from build123d import *

# Parameters (mm, degrees)
REVOLVE_2_ANGLE     = 180
EXTRUDE_3_REACH     = 142.262
SKETCH_1_12_R       = 4.474143501
CUT_EXTRUDE_3_DEPTH = 204.9
SKETCH_1_14_R       = 4.474143501
EXTRUDE_4_DEPTH     = 10
SKETCH_1_16_R       = 3
CUT_EXTRUDE_4_DEPTH = 32


with BuildPart() as part:
    # Sketch 1 → Revolve 2 (revolve)
    with BuildSketch(Plane.XY):
        Polygon((14, 48.5), (10, 48.5), (10, 32), (7, 32), (7, 35), (0, 35), (0, 51), (14, 51), (14, 52.5), (53.673378029, 34), (119, 34), (119, 32), (53.673378029, 32), align=None)
    revolve(axis=Axis((0, 0, 0), (1, 0, 0)), revolution_arc=REVOLVE_2_ANGLE)

    # Sketch 1_11 → Extrude 3 (add, up to next)
    with BuildSketch(Plane.XY, mode=Mode.PRIVATE) as extrude_3_sk1:
        Polygon((25, 43.925143786), (25, 32), (35, 32), (35, 39.766183592), align=None)
    extrude_3_tool1 = extrude(extrude_3_sk1.sketch, amount=EXTRUDE_3_REACH, mode=Mode.PRIVATE) - part.part
    extrude_3 = extrude_3_tool1.solids().sort_by_distance((29.647987, 36.996032, 0))[0]
    add(extrude_3)

    # Sketch 1_12 → Cut-Extrude 3 (cut)
    with BuildSketch(Plane.XY):
        with Locations(Location((30, 37, 0), (0, 0, 38.236616633))):
            Circle(SKETCH_1_12_R)
    cut_extrude_3 = extrude(amount=CUT_EXTRUDE_3_DEPTH, mode=Mode.SUBTRACT)

    # Sketch 1_14 → Extrude 4 (add)
    with BuildSketch(Plane.XY):
        with Locations(Location((30, 37, 0), (0, 0, 38.236616633))):
            Circle(SKETCH_1_14_R)
    extrude_4 = extrude(amount=EXTRUDE_4_DEPTH)

    # Sketch 1_16 → Cut-Extrude 4 (cut)
    with BuildSketch(Plane.XY):
        with Locations((30, 37)):
            Circle(SKETCH_1_16_R)
    cut_extrude_4 = extrude(amount=CUT_EXTRUDE_4_DEPTH, mode=Mode.SUBTRACT)

    # Mirror 1: Extrude 3, Cut-Extrude 3, Extrude 4, Cut-Extrude 4 across plane
    add(extrude_3.mirror(Plane.ZX))
    add(cut_extrude_3.mirror(Plane.ZX), mode=Mode.SUBTRACT)
    add(extrude_4.mirror(Plane.ZX))
    add(cut_extrude_4.mirror(Plane.ZX), mode=Mode.SUBTRACT)


solid = part.part
CAD build for the part. Positions are in the model's coordinates, mm. A direction names the side the tool comes from. Give positions to 0.01 mm unless a question says otherwise; leave off trailing zeros. Loops run counter-clockwise (first coordinate to the right, second up) from the corner with the lowest first, then second, coordinate; pieces in that order, holes last. Notation, with made-up numbers: M 23.25,-17 L 65.25,-17 A30 ccw 65.25,5 Z; hole C 12.25,50 d3. An arc over 180 degrees is marked long. One line per question, with ' | ' between items. Start each with the question number.
1. Two-plate mould, pull along Y, no slides. Class faces 6 (the face through (33, -38, 10)), 7 (the face through (37, 41, 0)), 8 (the face through (30, 32, 15)), 9 (the face through (86.79, 0.75, 33.99)): pulls with the +Y half, pulls with the -Y half, needs draft (parallel to the pull), parting line crosses it, or undercut.
2. Probe L1, parallel to X at y = 37, z = 4; L2, parallel to Y at x = 30, z = 4; L3, parallel to X at y = -37, z = 3.25. List the from-to ranges inside material, lowest first. Write a range as from..to.
3. Saw through at A-A on x = 30. Give the cut face in (y, z), plus the area to 3 significant figures.
4. 3-axis set-ups, long thin cutter, end or side, ignore diameter. For faces 1 (the face through (38.523, 0.903, 41.055)), 2 (the face through (25, 37, 11)), 3 (the face through (14, 0, 52)), 4 (the face through (3.45, 0.77, 34.99)), 5 (the face through (28.896, 32.664, 18.418)): which of +Z, -Z, +X, -X, +Y, -Y reach the whole face in a straight line?
5. Saw through at B-B on y = 0. Give the cut face in (x, z).
6. Saw through at C-C on x = 57. Give the cut face in (y, z), plus the area to 3 significant figures.
7. Flat gauge pins, fed straight in: pin 1 (1 mm diameter, centred on x = 66.5, z = 35, fed in from +Y); pin 2 (1.5 mm diameter, centred on x = 97, z = 20.5, fed in from +Y); pin 3 (7 mm diameter, centred on x = 30, y = 37, fed in from +Z); pin 4 (14.5 mm diameter, centred on x = 30, y = 37, fed in from -Z). Where does each tip first touch, or does it go through?
Result sheet:
1) face 6: undercut | face 7: needs draft | face 8: undercut | face 9: parting line crosses it
2) L1: x = 0..10, 25..27, 33..35, 41.13..46.78 | L2: y = -44.86..-40, -34..-32, 32..34, 40..44.86 | L3: x = 0..10, 25..27, 33..35, 41.31..46.93
3) outline: M -45.04,0 L -40,0 L -40,10 L -41.47,10 L -41.47,17.56 A45.04 ccw Z; M -34,0 L -32,0 L -32,26.96 A41.85 cw 32,26.96 L 32,0 L 34,0 L 34,10 L 32.53,10 L 32.53,31.15 A45.04 ccw -32.53,31.15 L -32.53,10 L -34,10 Z; M 40,0 L 45.04,0 A45.04 ccw 41.47,17.56 L 41.47,10 L 40,10 Z | area: 406 mm^2
4) face 1: +Z, +X | face 2: -Z | face 3: +Z, -X | face 4: -Z, -X | face 5: +Z
5) outline: M 0,35 L 7,35 L 7,32 L 10,32 L 10,48.5 L 14,48.5 L 53.67,32 L 119,32 L 119,34 L 53.67,34 L 14,52.5 L 14,51 L 0,51 Z
6) outline: M -34,0 L -32,0 A32 cw 32,0 L 34,0 A34 ccw Z | area: 207 mm^2
7) pin 1: passes through | pin 2: stops at y = 27.68 | pin 3: stops at z = 10 | pin 4: stops at z = 0
